```python
from build123d import *

# Parameters (mm, degrees)
EXTRUDE_1_DEPTH          = 17.5
SKETCH_2_OUTSIDE_W       = 142.004
SKETCH_2_OUTSIDE_H       = 141.066
SKETCH_2_OUTSIDE_R       = 3.031088913
CUT_EXTRUDE_1_DEPTH      = 36.304921753
CUT_EXTRUDE_1_DRAFT      = -60
HOLE_WIZARD_M3_1_D       = 2.5
HOLE_WIZARD_M3_2_D       = 2.5
MIRROR_1_COPY_1_SKETCH_W = 142.004
MIRROR_1_COPY_1_SKETCH_H = 141.066
MIRROR_1_COPY_1_SKETCH_R = 3.031088913
MIRROR_1_COPY_1_DEPTH    = 36.304921753
MIRROR_1_COPY_1_DRAFT    = -60
CHAMFER_1_SIZE           = 0.2


with BuildPart() as part:
    # 草图1 → 凸台-拉伸1 (new, symmetric)
    with BuildSketch(Plane.XY):
        Polygon((3.5, 0), (1.75, 3.031088913), (-1.75, 3.031088913), (-3.5, 0), (-1.75, -3.031088913), (1.75, -3.031088913), align=None)
    extrude(amount=EXTRUDE_1_DEPTH, both=True)


with BuildPart() as cut_extrude_1_tool:
    # 草图2 outside → 切除-拉伸1 (with draft: the straight prism first)
    with BuildSketch(Plane.XY.offset(17.5)):
        Rectangle(SKETCH_2_OUTSIDE_W, SKETCH_2_OUTSIDE_H)
        Circle(SKETCH_2_OUTSIDE_R, mode=Mode.SUBTRACT)
    extrude(amount=-CUT_EXTRUDE_1_DEPTH)
    # 切除-拉伸1: the draft: its side faces are tilted about the plane it starts from
    cut_extrude_1_sides = [cut_extrude_1_tool.faces().sort_by_distance(p)[0] for p in [
        (0, -70.533, -0.652460877),
        (71.002, 0, -0.652460877),
        (0, 70.533, -0.652460877),
        (-71.002, 0, -0.652460877),
        (-3.031088913, 0, -0.652460877),
    ]]
    draft(cut_extrude_1_sides, Plane.XY.offset(17.5), CUT_EXTRUDE_1_DRAFT)


with BuildPart() as part_1:
    add(part.part)

    # 切除-拉伸1: cut by cut_extrude_1_tool
    add(cut_extrude_1_tool.part, mode=Mode.SUBTRACT)

    # M3 螺纹孔1 (through all)
    with Locations(Plane.XY.offset(17.5)):
        with Locations((0, 0)):
            hole_wizard_m3_1 = Hole(HOLE_WIZARD_M3_1_D / 2)

    # M3 螺纹孔2 (through all)
    with Locations(Plane(origin=(0, 3.031088913, 0), x_dir=(1, 0, 0), z_dir=(0, 1, 0))):
        with Locations((0, -9.5)):
            hole_wizard_m3_2 = Hole(HOLE_WIZARD_M3_2_D / 2)

    # 镜向1: M3 螺纹孔1, M3 螺纹孔2 across plane
    add(hole_wizard_m3_1.mirror(Plane.XY), mode=Mode.SUBTRACT)
    add(hole_wizard_m3_2.mirror(Plane.XY), mode=Mode.SUBTRACT)


with BuildPart() as mirror_1_copy_1_tool:
    # 镜向1 copy 1 sketch → 镜向1 copy 1 (with draft: the straight prism first)
    with BuildSketch(Plane(origin=(0, 0, -17.5), x_dir=(1, 0, 0), z_dir=(0, 0, -1))):
        Rectangle(MIRROR_1_COPY_1_SKETCH_W, MIRROR_1_COPY_1_SKETCH_H)
        Circle(MIRROR_1_COPY_1_SKETCH_R, mode=Mode.SUBTRACT)
    extrude(amount=-MIRROR_1_COPY_1_DEPTH)
    # 镜向1 copy 1: the draft: its side faces are tilted about the plane it starts from
    mirror_1_copy_1_sides = [mirror_1_copy_1_tool.faces().sort_by_distance(p)[0] for p in [
        (0, -70.533, 0.652460877),
        (71.002, 0, 0.652460877),
        (0, 70.533, 0.652460877),
        (-71.002, 0, 0.652460877),
        (-3.031088913, 0, 0.652460877),
    ]]
    draft(mirror_1_copy_1_sides, Plane(origin=(0, 0, -17.5), x_dir=(1, 0, 0), z_dir=(0, 0, -1)), MIRROR_1_COPY_1_DRAFT)


with BuildPart() as part_2:
    add(part_1.part)

    # 镜向1 copy 1: cut by mirror_1_copy_1_tool
    add(mirror_1_copy_1_tool.part, mode=Mode.SUBTRACT)

    # 倒角1
    chamfer_1_edges = [part_2.edges().sort_by_distance(p)[0] for p in [
        (1.25, -3.031088913, -9.5),
        (1.25, 3.031088913, -9.5),
        (1.25, 0, 17.5),
        (1.25, 0, -17.5),
        (1.25, -3.031088913, 9.5),
        (1.25, 3.031088913, 9.5),
    ]]
    chamfer(chamfer_1_edges, length=CHAMFER_1_SIZE)


solid = part_2.part
```
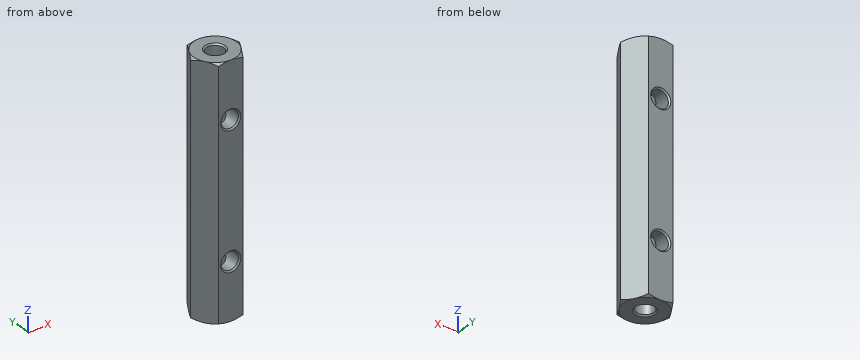
The listing builds one solid part. Answer for the finished solid, in the listing's coordinates (mm). Coordinates: 2 decimals unless noted, no trailing zeros. Write each loop counter-clockwise with the first axis right and the second up, starting at its lowest first coordinate (ties: lowest second). Pieces come first, ordered by that corner, then holes. Notation, with made-up numbers: (68, -28) - (112, -28) arc R28 ccw to (112, -10) - close; hole circle Ø3 at (70.5, 7.25). An arc over 180 degrees is marked (long way). Return JSON: item names as keys, results as strings. Group by question number.
Q1. Flat-ended cylindrical pins translate along their axes: pin 1 Ø2 at (y, z) = (-1.5, 4) entering from +X; pin 2 Ø2 at (y, z) = (-0.5, 6.5) entering from +X; pin 3 Ø1 at (x, z) = (2.5, 9) entering from +Y; pin 4 Ø3 at (x, z) = (0, -9.5) entering from -Y. Find the tip coordinate at first contact, or state that the pin passes through.
Q2. The part is cut by section B-B on x = -0.5. State how many separate pieces and enclosed holes the cut face has, and give its area (3 significant figures).
Q3. The part is cut by section A-A on z = 4. Write down the section's boundary in (x, y), and give its area (3 significant figures).
Q4. Find the intervals of material crossed by line 1 along Z through (x, y) = (0, 1.45); line 2 along Y through (x, z) = (0, -4.25); line 3 along Z through (x, y) = (0.5, 2.5), in increasing order. Write a range as [from, to].
Evaluation:
{
 "1": {"pin 1": "stops at x = 3.21", "pin 2": "stops at x = 3.5", "pin 3": "stops at y = 2.6", "pin 4": "stops at y = -3.03"},
 "2": {"separate pieces": "6", "enclosed holes": "0", "area": "114 mm2"},
 "3": {"outline": "(-3.5, 0) - (-1.75, -3.03) - (1.75, -3.03) - (3.5, 0) - (1.75, 3.03) - (-1.75, 3.03) - close; hole circle Ø2.5 at (0, 0)", "area": "26.9 mm2"},
 "4": {"line 1": "z = [-17.5, -10.75], [-8.25, 8.25], [10.75, 17.5]", "line 2": "y = [-3.03, -1.25], [1.25, 3.03]", "line 3": "z = [-17.5, -10.65], [-8.35, 8.35], [10.65, 17.5]"}
}
